Autodesk Inventor part; units mm, degrees
ref_plane "YZ Plane" through (0, 0, 0) normal (1, 0, 0) x (0, 1, 0)
ref_plane "XZ Plane" through (0, 0, 0) normal (0, 1, 0) x (-1, 0, 0)
ref_plane "XY Plane" through (0, 0, 0) normal (0, 0, 1) x (1, 0, 0)
sketch "Sketch2" plane through (0, 0, 0) normal (0, 0, 1) x (1, 0, 0)
  line L0 (-64.4682, 0) -> (-70.3341, -10.16)
  line L1 (-70.3341, -10.16) -> (-82.0659, -10.16)
  line L2 (-82.0659, -10.16) -> (-87.9318, 0)
  line L3 (-87.9318, 0) -> (-82.0659, 10.16)
  line L4 (-82.0659, 10.16) -> (-70.3341, 10.16)
  line L5 (-70.3341, 10.16) -> (-64.4682, 0)
  line L6 (-76.2, 0) -> (76.2, 0) construction
  line L7 (82.0659, -10.16) -> (70.3341, -10.16)
  line L8 (70.3341, -10.16) -> (64.4682, 0)
  line L9 (64.4682, 0) -> (70.3341, 10.16)
  line L10 (70.3341, 10.16) -> (82.0659, 10.16)
  line L11 (82.0659, 10.16) -> (82.4325, 9.525)
  line L12 (-132.627, 0) -> (135.7899, 0)
  line L13 (0, 0) -> (0, 37.2208) construction
  line L14 (0, 9.525) -> (30.7487, 9.525)
  line L15 (0, 9.525) -> (-30.7487, 9.525)
  circle A0 centre (-76.2, 0) radius 18.0818
  line L16 (-87.9318, 0) -> (-94.2818, 0) construction
  arc A1 (61.0244, 14.8673) -> (61.0244, -14.8673) centre (76.2, 0) ccw
  line L17 (87.9318, 0) -> (97.4446, 0) construction
  line L18 (87.9318, 0) -> (89.9839, -16.166) construction
  line L19 (30.7487, 9.525) -> (70.3341, 16.51)
  line L20 (-76.2, 18.0818) -> (-30.7487, 9.525)
  line L21 (70.3341, 10.16) -> (70.3341, 16.51) construction
  line L22 (82.0659, 10.16) -> (82.0659, 16.51)
  line L23 (82.0659, -10.16) -> (82.0659, -16.51)
  line L24 (0, -9.525) -> (30.7487, -9.525)
  line L25 (0, -9.525) -> (-30.7487, -9.525)
  line L26 (30.7487, -9.525) -> (70.3341, -16.51)
  line L27 (-76.2, -18.0818) -> (-30.7487, -9.525)
  line L28 (70.3341, 16.51) -> (82.0659, 16.51)
  line L29 (70.3341, -10.16) -> (70.3341, -16.51) construction
  line L30 (70.3341, -16.51) -> (82.0659, -16.51)
  point P0 (82.0659, 18.5801)
  point P1 (82.0659, -18.5801)
  dimension "centerToBoxEndWrench" = 76.2
  dimension "boltPrintedSize" = 20.32
  dimension "centerToOpenEndWrench" = 76.2
  dimension "d23" = 9.525
  dimension "d24" = 6.35
  dimension "d26" = 6.35
extrude "Extrusion2" add sketch "Sketch2" along normal mid plane 6.35 contours L12 A0 L27 L2 L1 L0 | L5 L4 L3 L12 A0 L20 | A0 L20 L15 L14 L19 A1 L12 | L12 A1 L26 L24 L25 L27 A0 | A1 L19 L28 L22 L10 L9 L12 | L12 L8 L7 L23 L30 L26 A1
fillet "Fillet1" radius 0.7937 4 edges at (82.0659, 16.51, 0) (82.0659, 10.16, 0) (82.0659, -10.16, 0) (82.0659, -16.51, 0)
fillet "Fillet2" radius 6.35 8 edges at (-30.7487, -9.525, 0) (30.7487, -9.525, 0) (70.3341, -16.51, 0) (-76.2, -18.0818, 0) (-76.2, 18.0818, 0) (-30.7487, 9.525, 0) (30.7487, 9.525, 0) (70.3341, 16.51, 0)
equation "\"centerToBoxEndWrench\" = 4 * boltSize"
equation "\"boltPrintedSize\" = boltSize + boltGap"
equation "\"centerToOpenEndWrench\" = 4 * boltSize"
equation "\"d23\" = 0.5 * boltSize"
equation "\"d24\" = minWallThickness"
equation "\"d26\" = minWallThickness"
equation "\"d27\" = minWallThickness"
equation "\"minWallThickness\" = 6.35"
equation "\"boltGap\" = 1.27"
equation "\"boltSize\" = 19.05"
properties part number "3_4_inchWrenchV04"
The listing builds one solid part. Answer for the finished solid, in the listing's coordinates (mm). A direction names the side the tool comes from. Give positions to 0.01 mm unless a question says otherwise; leave off trailing zeros. Order: outer loops, then holes, each group sorted by start corner. A loop starts at its lowest first (then second) coordinate and runs counter-clockwise, first axis right, second up. Notation, with made-up numbers: (-0.5, 12.5) -> (44.5, 12.5) arc R24 ccw to (44.5, 32.5) -> close; hole circle Ø7 at (76, -33.5). An arc over 180 degrees is marked (long way). Put each result on its own line as item: value.
Item 1: For faces 1 (the face through (-76, 10.16, 0)), 2 (the face through (76, -16.51, 0)), 3 (the face through (67.44, -5.15, -0.04)), determine the directions among +Z, -Z, +X, -X, +Y, -Y from which every point of the face is accessible in a straight line to the end or side of a thin tool.
Established:
face 1: +Z, -Z
face 2: +Z, -Z, +X, -Y
face 3: +Z, -Z, +X
Item 2: A cutting plane is placed at D-D on x = 24.5. Give the vertices of the cut face in (y, z) (3 decimals), plus the area to 3 significant figures.
Established:
outline: (-9.525, -3.175) -> (9.525, -3.175) -> (9.525, 3.175) -> (-9.525, 3.175) -> close
area: 121 mm^2
Item 3: A cutting plane is placed at C-C on x = -73. Give the vertices of the cut face in (y, z) (3 decimals), plus the area to 3 significant figures.
Established:
outline: (-17.479, -3.175) -> (-10.16, -3.175) -> (-10.16, 3.175) -> (-17.479, 3.175) -> close; (10.16, -3.175) -> (17.479, -3.175) -> (17.479, 3.175) -> (10.16, 3.175) -> close
area: 93.0 mm^2
Item 4: For a pull along Y with two mould halves and no side action, classify faces 4 (the face through (-7, 0, -3.175)), 5 (the face through (-53.752, 13.856, -0.044)), 6 (the face through (76, 10.16, 0)) as released by +Y, released by -Y, zero draft, split by the parting line, or undercut.
Established:
face 4: zero draft
face 5: released by +Y
face 6: undercut
Item 5: A cutting plane is placed at B-B on y = 12.5. Give the vertices of the cut face in (x, z) (3 decimals), plus the area to 3 significant figures.
Established:
outline: (-89.265, -3.175) -> (-46.551, -3.175) -> (-46.551, 3.175) -> (-89.265, 3.175) -> close; (47.609, -3.175) -> (82.066, -3.175) -> (82.066, 3.175) -> (47.609, 3.175) -> close
area: 490 mm^2
Item 6: Given P1, Ø1.9, axis at x = 74, z = -0.5, coming from the +Y side; P2, Ø1.9, axis at x = 76.5, z = 1, coming from the -Y side; P3, Ø3, axis at x = 6.5, z = 0, coming from the -Y side (3 decimals), each flat-ended and moving along its own axis, determine where each tip first touches the part or whether it passes through.
Established:
P1: stops at y = 16.51
P2: stops at y = -16.51
P3: stops at y = -9.525
Item 7: Straight lines are drawn through the part: line 1 (Y direction, x = -30.5, z = 1.5); line 2 (Y direction, x = -79.5, z = 2.75); line 3 (X direction, y = -7, z = 2.5). For each, find the intervals that lie inside material, in ascending order.
Established:
line 1: y = -9.53 to 9.53
line 2: y = -17.78 to -10.16, 10.16 to 17.78
line 3: x = -92.87 to -83.89, -68.51 to 68.51
